For this review, take the finished solid that the model builds, in its own axes (mm). Face numbers are marked on the shaded views. A direction names the side the tool comes from. Give positions to 0.01 mm unless a question says otherwise; leave off trailing zeros. Write each loop counter-clockwise with the first axis right and the second up, starting at its lowest first coordinate (ties: lowest second). Pieces come first, ordered by that corner, then holes.
Q1. We need section D-D (z = 55). Write out the cut boundary in (x, y) (1 decimal), then the cut area to 3 significant figures.
Q2. For line 1 (X direction, y = -30, z = 77); line 2 (Y direction, x = 88, z = 58); line 3 (X direction, y = -18, z = 48), list the stretches that pass through material, from the lowest coordinate up.
Q3. Mouldability with a two-part tool opening along Y and no side actions: class the marked faces 1, 2, 3 and 4 as released by +Y, released by -Y, zero draft, split by the parting line, or undercut.
Q4. Insertion check: P1, Ø5, axis at y = -22, z = 54, coming from the +X side; P2, Ø5, axis at y = -13, z = 56, coming from the -X side; P3, Ø17.5, axis at x = 54.5, y = -13.5, coming from the +Z side; P4, Ø14.5, axis at x = 31.12, y = -18.07, coming from the +Z side. Each pin has a flat end and moves straight along its axis. Give the tip position at first contact, or say it passes through.
Q5. Machinability: for the marked faces 5, 6, 7, 8 and 9, which of the approach directions +Z, -Z, +X, -X, +Y, -Y give a long, thin tool a straight path to every point of the face, cutting with its end or side? Answer none if there is none.
Q6. We need section A-A (z = 75). Write out the cut boundary in (x, y), then the cut area to 3 significant figures.
Q7. We need section B-B (x = 77). Write out the cut boundary in (y, z), then the cut area to 3 significant figures.
```python
from build123d import *

# Parameters (mm, degrees)
F0_W     = 31.75
F0_H     = 31.75
F0_R     = 15.875
F0_H_2   = 28.8293883204
F1_DEPTH = 31.75
F0_H_3   = 91.8206116796
F0_H_4   = 94.7412233591
F2_DEPTH = 73.025
F3_DEPTH = 92.075
F4_DEPTH = 22.225
F5_SCALE = 0.5


with BuildPart() as f1:
    # F0 (on Top) → F1 (new body)
    with BuildSketch(Plane.XY):
        Polygon((-114.9314489663, -5.3708956957), (-114.9314489663, -56.1708956957), (-57.7814489663, -56.1708956957), (-57.7814489663, -24.4208956957), (-57.7814489663, 67.3997159839), (-57.7814489663, 96.2291043043), (-114.9314489663, 96.2291043043), (-114.9314489663, 45.4291043043), (-73.6564489663, 45.4291043043), (-73.6564489663, -5.3708956957), align=None)
        with Locations((-41.9064489663, -40.2958956957)):
            Rectangle(F0_W, F0_H)
        Polygon((-26.0314489663, -24.4208956957), (-26.0314489663, -56.1708956957), (50.1685510337, -56.1708956957), (50.1685510337, -27.3415073752), (50.1685510337, 67.3997159839), (50.1685510337, 96.2291043043), (-26.0314489663, 96.2291043043), (-26.0314489663, 67.3997159839), align=None)
        with Locations((12.0685510337, 20.0291043043)):
            Circle(F0_R, mode=Mode.SUBTRACT)
        with Locations((66.0435510337, -41.7562015355)):
            Rectangle(F0_W, F0_H_2)
        with Locations((-41.9064489663, 81.8144101441)):
            Rectangle(F0_W, F0_H_2)
        Polygon((81.9185510337, -27.3415073752), (81.9185510337, -56.1708956957), (139.0685510337, -56.1708956957), (139.0685510337, -5.3708956957), (97.7935510337, -5.3708956957), (97.7935510337, 45.4291043043), (139.0685510337, 45.4291043043), (139.0685510337, 96.2291043043), (81.9185510337, 96.2291043043), (81.9185510337, 67.3997159839), align=None)
        with Locations((66.0435510337, 81.8144101441)):
            Rectangle(F0_W, F0_H_2)
    extrude(amount=F1_DEPTH)

    # F0 (on Top) → F2 (join)
    with BuildSketch(Plane.XY):
        with Locations((-41.9064489663, 21.4894101441)):
            Rectangle(F0_W, F0_H_3)
        with Locations((66.0435510337, 20.0291043043)):
            Rectangle(F0_W, F0_H_4)
    extrude(amount=F2_DEPTH)

    # F0 (on Top) → F3 (join)
    with BuildSketch(Plane.XY):
        with Locations((-41.9064489663, 81.8144101441)):
            Rectangle(F0_W, F0_H_2)
        with Locations((-41.9064489663, -40.2958956957)):
            Rectangle(F0_W, F0_H)
        with Locations((66.0435510337, -41.7562015355)):
            Rectangle(F0_W, F0_H_2)
        with Locations((66.0435510337, 81.8144101441)):
            Rectangle(F0_W, F0_H_2)
    extrude(amount=F3_DEPTH)

    # F4 (add): a face of the model
    f4_faces = [f1.faces().sort_by_distance(p)[0] for p in [
        (-24.3275651674, 20.0291043043, 31.75),
    ]]
    extrude(f4_faces, amount=F4_DEPTH)


with BuildPart() as f1_1:
    # F5: moved
    add(f1.part.scale(F5_SCALE).moved(Location((25.0842755169, -28.0854478478, 46.0375))))


solid = f1_1.part
```
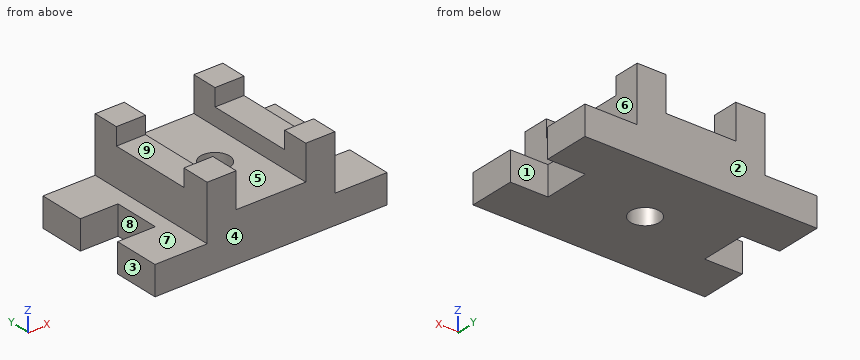
Computed:
1. outline: (-32.4, -56.2) - (94.6, -56.2) - (94.6, -30.8) - (74, -30.8) - (74, -5.4) - (94.6, -5.4) - (94.6, 20) - (-32.4, 20) - (-32.4, -5.4) - (-11.7, -5.4) - (-11.7, -30.8) - (-32.4, -30.8) - close; hole circle Ø15.9 at (31.1, -18.1)
1. area: 8,430 mm2
2. line 1: x = -3.81 to 12.07, 50.17 to 66.04
2. line 2: y = -56.17 to -30.77, -5.37 to 20.03
2. line 3: x = -11.74 to 23.18, 39.06 to 73.98
3. face 1: undercut
3. face 2: released by +Y
3. face 3: zero draft
3. face 4: released by -Y
4. P1: stops at x = 73.98
4. P2: stops at x = -11.74
4. P3: stops at z = 82.55
4. P4: passes through
5. face 5: +Z, +Y, -Y
5. face 6: +Z, +X, +Y, -Y
5. face 7: +Z, -X, +Y, -Y
5. face 8: +Z, -Z, -X
5. face 9: +Z, +X, -X
6. outline: (-3.81, -56.17) - (12.07, -56.17) - (12.07, 20.03) - (-3.81, 20.03) - close; (50.17, -56.17) - (66.04, -56.17) - (66.04, 20.03) - (50.17, 20.03) - close
6. area: 2,420 mm2
7. outline: (-56.17, 46.04) - (-30.77, 46.04) - (-30.77, 61.91) - (-56.17, 61.91) - close; (-5.37, 46.04) - (20.03, 46.04) - (20.03, 61.91) - (-5.37, 61.91) - close
7. area: 806 mm2
